Geometry check sheet. Reference: the model listing, model coordinates, mm. A direction names the side the tool comes from. Round coordinates to 2 decimals unless told otherwise and drop trailing zeros. Write each loop counter-clockwise with the first axis right and the second up, starting at its lowest first coordinate (ties: lowest second). Pieces come first, ordered by that corner, then holes. Notation, with made-up numbers: M 64,20 L 92,20 A18 cw 92,37 Z; hole C 70.5,25 d5. An arc over 180 degrees is marked long. Use a Markdown table: item, result.
```python
from build123d import *

# Parameters (mm, degrees)
F1_DEPTH = 10
F2_R     = 5
F3_R     = 2.75
F4_DEPTH = 20
F6_DEPTH = 3.5


with BuildPart() as f1:
    # F0 (on Front) → F1 (new body, symmetric)
    with BuildSketch(Plane.XZ):
        with BuildLine():
            Line((-5.4335961189, 15.0491206792), (0, 0))
            Line((0, 0), (40, 0))
            Line((40, 0), (40, 3.5))
            Line((40, 3.5), (23.5106382979, 3.5))
            ThreePointArc((23.5106382979, 3.5), (20.6374861905, 4.4079348774), (18.8077880856, 6.8020012129))
            Line((18.8077880856, 6.8020012129), (13.3778047301, 21.8411158278))
            Line((13.3778047301, 21.8411158278), (10.0858095816, 20.6525166768))
            Line((10.0858095816, 20.6525166768), (13.3120072771, 11.7171012735))
            Line((13.3120072771, 11.7171012735), (1.0845967253, 7.3023044269))
            Line((1.0845967253, 7.3023044269), (-2.1416009703, 16.2377198302))
            Line((-2.1416009703, 16.2377198302), (-5.4335961189, 15.0491206792))
        make_face()
    extrude(amount=F1_DEPTH, both=True)

    # F2
    f2_edges = [f1.edges().sort_by_distance(p)[0] for p in [
        (-3.787599, 10, 15.64342),
        (11.731807, 10, 21.246816),
        (11.731807, -10, 21.246816),
        (-3.787599, -10, 15.64342),
        (40, -10, 1.75),
        (40, 10, 1.75),
    ]]
    fillet(f2_edges, radius=F2_R)

    # F3 (on face) → F4 (cut, through all)
    with BuildSketch(Plane(origin=(18.811400849, 0, 6.7919951486), x_dir=(0, 1, 0), z_dir=(0.9405700424, 0, 0.3395997574))):
        with Locations((0, 11.25)):
            Circle(F3_R)
    extrude(amount=-F4_DEPTH, mode=Mode.SUBTRACT)

    # F5 (on face) → F6 (cut, through all)
    with BuildSketch(Plane.XY.offset(3.5)):
        with BuildLine():
            ThreePointArc((28.5106382979, -3), (30.6319586414, -2.1213203436), (31.5106382979, 0))
            ThreePointArc((31.5106382979, 0), (30.6319586414, 2.1213203436), (28.5106382979, 3))
            ThreePointArc((28.5106382979, 3), (25.5106382979, 0), (28.5106382979, -3))
        make_face()
        with BuildLine():
            ThreePointArc((28.5106382979, 3), (30.6319586414, 2.1213203436), (31.5106382979, 0))
            ThreePointArc((31.5106382979, 0), (30.6319586414, -2.1213203436), (28.5106382979, -3))
            Line((28.5106382979, -3), (40, -3))
            Line((40, -3), (40, 3))
            Line((40, 3), (28.5106382979, 3))
        make_face()
    extrude(amount=-F6_DEPTH, mode=Mode.SUBTRACT)


solid = f1.part
```
Item 1: Cross-section at C-C, the plane y = 2. Record the cut outline in (x, z), and give its area (3 significant figures).
Outcome:
| item | result |
|---|---|
| outline | M -5.43,15.05 L -4.46,12.36 L -1.17,13.55 L -2.14,16.24 Z; M -3.18,8.81 L 0,0 L 26.27,0 L 26.27,3.5 L 23.51,3.5 A5 cw 18.81,6.8 L 15.63,15.6 L 12.34,14.41 L 13.31,11.72 L 1.08,7.3 L 0.11,9.99 Z; M 10.09,20.65 L 11.06,17.96 L 14.35,19.15 L 13.38,21.84 Z |
| area | 264 mm2 |
Item 2: Mould release check, pull along Z, two halves, no side actions. Record for faces 5 (the face through (34, 3, 2)), 6 (the face through (-3.077, -0.358, 13.749)), 7 (the face through (12.193, -8.496, 19.897)): +Z half, -Z half, draft (parallel to the pull), parting line (faces both ways), or undercut.
Outcome:
| item | result |
|---|---|
| face 5 | draft |
| face 6 | undercut |
| face 7 | +Z half |
Item 3: Cross-section at A-A, the plane x = 33. Record the cut outline in (y, z), and give its area (3 significant figures).
Outcome:
| item | result |
|---|---|
| outline | M -10,0 L -3,0 L -3,3.5 L -10,3.5 Z; M 3,0 L 10,0 L 10,3.5 L 3,3.5 Z |
| area | 49.0 mm2 |
Item 4: Material ranges on line 1 along Z through (x, y) = (38.5, 8); line 2 along Y through (x, z) = (29, 1.5); line 3 along X through (y, z) = (-2.25, 4.5), recorded low to high. Write a range as from..to.
Outcome:
| item | result |
|---|---|
| line 1 | z = 0..3.5 |
| line 2 | y = -10..-3, 3..10 |
| line 3 | x = -1.62..20.51 |
Item 5: Go/stop test with flat-tipped pins: pin 1 (2 mm diameter, centred on x = 7, y = 1.5, fed in from -Z); pin 2 (1.5 mm diameter, centred on y = 1, z = 13, fed in from +X); pin 3 (1 mm diameter, centred on x = 3, y = -7, fed in from +Z); pin 4 (1 mm diameter, centred on y = -5.5, z = 11.5, fed in from +X). Record where each tip stops, or that it passes through.
Outcome:
| item | result |
|---|---|
| pin 1 | stops at z = 0 |
| pin 2 | stops at x = 16.84 |
| pin 3 | stops at z = 8.17 |
| pin 4 | stops at x = 17.29 |
Item 6: Cross-section at B-B, the plane y = 0. Record the cut outline in (x, z) (3 decimals).
Outcome:
| item | result |
|---|---|
| outline | M -5.434,15.049 L -4.754,13.168 L -1.462,14.357 L -2.142,16.238 Z; M -2.887,7.995 L 0,0 L 25.511,0 L 25.511,3.5 L 23.511,3.5 A5 cw 18.808,6.802 L 15.925,14.787 L 12.633,13.598 L 13.312,11.717 L 1.085,7.302 L 0.405,9.183 Z; M 10.086,20.653 L 10.765,18.771 L 14.057,19.96 L 13.378,21.841 Z |
Item 7: Cross-section at D-D, the plane y = 8.75. Record the cut outline in (x, z).
Outcome:
| item | result |
|---|---|
| outline | M -4.86,13.46 L 0,0 L 38.31,0 L 38.31,3.5 L 23.51,3.5 A5 cw 18.81,6.8 L 13.95,20.25 L 10.66,19.06 L 13.31,11.72 L 1.08,7.3 L -1.57,14.65 Z |
Item 8: Access from +Z, -Z, +X, -X, +Y, -Y to the whole of each face (thin tool, end or side, straight path). Record for faces 1 (the face through (32, -5, 3.5)), 2 (the face through (34, -3, 2)), 3 (the face through (0.21, 2.08, 9.72)), 4 (the face through (-3.3, 8.5, 14.3)).
Outcome:
| item | result |
|---|---|
| face 1 | +Z, +X, +Y, -Y |
| face 2 | +Z, -Z, +X |
| face 3 | +Z, +Y, -Y |
| face 4 | +Z, -X, +Y |
